Autodesk Inventor part; units mm, degrees
ref_plane "Work Plane2" through (0, 0, 16.5) normal (0, 0, 1) x (1, 0, 0)
ref_plane "YZ Plane" through (0, 0, 0) normal (1, 0, 0) x (0, 1, 0)
ref_plane "XZ Plane" through (0, 0, 0) normal (0, 1, 0) x (-1, 0, 0)
sketch "Sketch1" plane through (0, 0, 0) normal (0, 1, 0) x (-1, 0, 0)
  circle A0 centre (0, 0) radius 25
  dimension "d12" = 50
extrude "Extrusion1" add sketch "Sketch1" along normal blind 2
mirror "Mirror1" about plane through (0, 0, 0) normal (0, 0, 1)
ref_plane "Work Plane2" through (0, 0, 16.5) normal (0, 0, 1) x (1, 0, 0)
sketch "Sketch9" plane through (0, 0, 16.5) normal (0, 0, 1) x (1, 0, 0)
  line L0 (-5.099, 2) -> (5, 2)
  line L1 (5, 2) -> (5, 21)
  line L2 (-5.099, 20) -> (-5.099, 2)
  line L3 (0, -1.6) -> (0, 30.6) construction
  arc A0 (5, 21) -> (-5.099, 20) centre (0, 20) ccw
  circle A1 centre (0, 20) radius 1.9
  line L4 (25, 2) -> (-25, 2)
  dimension "d19" = 5
  dimension "d20" = 3.8
  dimension "d65" = 0
  dimension "d66" = 18
extrude "Extrusion3" add sketch "Sketch9" against normal blind 3
sketch "Sketch20" plane through (0, 0, 16.5) normal (0, 0, 1) x (1, 0, 0)
  circle A0 centre (0, 20) radius 1.9
  line L0 (-1.9, 20) -> (1.9, 20)
  line L1 (1.9, 20) -> (1.9, 25.4725)
  line L2 (1.9, 25.4725) -> (-1.9, 25.4725)
  line L3 (-1.9, 25.4725) -> (-1.9, 20)
  point P0 (0, 0)
extrude "Extrusion14" cut sketch "Sketch20" against normal blind 3 contours A0 L3 L2 L1
mirror "Mirror5" about plane through (0, 0, 0) normal (0, 0, 1) of "Extrusion3", "Extrusion14"
sketch "Sketch21" plane through (0, 0, 0) normal (0, -1, 0) x (1, 0, 0)
  circle A0 centre (0, 0) radius 16.95
  dimension "d62" = 33.9
extrude "Extrusion15" add sketch "Sketch21" along normal blind 30
ref_plane "Work Plane1" through (0, 0, 0) normal (0, 0, 1) x (1, 0, 0)
properties part number "BaseComple"
CAD build for the part. Positions are in the model's coordinates, mm. A direction names the side the tool comes from. Give positions to 0.01 mm unless a question says otherwise; leave off trailing zeros. Loops run counter-clockwise (first coordinate to the right, second up) from the corner with the lowest first, then second, coordinate; pieces in that order, holes last. Notation, with made-up numbers: (-32.75, 78) -> (-6.75, 78) arc R27 cw to (-6.75, 96) -> close; hole circle Ø11 at (40.5, 59). An arc over 180 degrees is marked (long way). Use a Markdown table: item, result.
1. Slice it at D-D (y = -22.5). List the corners of the cut face in (x, z).
Check result:
| item | result |
|---|---|
| outline | circle Ø33.9 at (0, 0) |
2. Flat gauge pins, fed straight in: pin 1 (2.5 mm diameter, centred on y = 8.5, z = 14.5, fed in from +X); pin 2 (0.9 mm diameter, centred on y = 22.5, z = 15.5, fed in from +X); pin 3 (10 mm diameter, centred on x = 12.5, z = -5, fed in from +Y). Where does each tip first touch, or does it go through?
Check result:
| item | result |
|---|---|
| pin 1 | stops at x = 5 |
| pin 2 | stops at x = 4.67 |
| pin 3 | stops at y = 2 |
3. Mould opens along Z. For faces 6 (the flat face through (-1.9, 22, 15)), 7 (the flat face through (0, 14, 16.5)), 8 (the flat face through (0, 14, 13.5)), 9 (the flat face through (0, 14, -16.5)) say: pulls with the +Z half, pulls with the -Z half, needs draft (parallel to the pull), parting line crosses it, or undercut.
Check result:
| item | result |
|---|---|
| face 6 | needs draft |
| face 7 | pulls with the +Z half |
| face 8 | undercut |
| face 9 | pulls with the -Z half |
4. Wall check: L1, parallel to Y at x = 19, z = -10.5; L2, parallel to Y at x = -8.5, z = -7; L3, parallel to X at y = 17, z = -14.5. Give the ranges that are in metal, low to high. Write a range as [from, to].
Check result:
| item | result |
|---|---|
| L1 | y = [0, 2] |
| L2 | y = [-30, 2] |
| L3 | x = [-5.1, 5] |
5. Slice it at C-C (x = -12.5). List the corners of the cut face in (y, z), plus the area to 3 significant figures.
Check result:
| item | result |
|---|---|
| outline | (-30, -11.45) -> (0, -11.45) -> (0, -21.65) -> (2, -21.65) -> (2, 21.65) -> (0, 21.65) -> (0, 11.45) -> (-30, 11.45) -> close |
| area | 773 mm^2 |
6. Which spindle directions (+Z, -Z, +X, -X, +Y, -Y) get a long thin tool onto all of the face, cutting with end or side? Do faces 1 (the cylindrical face through (-12.49, -14.79, -11.46)), 2 (the flat face through (5, 11, 15)), 3 (the flat face through (1.9, 22, -15)), 4 (the flat face through (-5.099, 11, -15)), 5 (the flat face through (0, -30, 0)). Say none if no direction does.
Check result:
| item | result |
|---|---|
| face 1 | -Y |
| face 2 | +Z, -Z, +X, +Y |
| face 3 | +Z, -Z, +Y |
| face 4 | +Z, -Z, -X, +Y |
| face 5 | +Z, -Z, +X, -X, -Y |
7. Slice it at B-B (x = 0). List the corners of the cut face in (y, z), plus the area to 3 significant figures.
Check result:
| item | result |
|---|---|
| outline | (-30, -16.95) -> (0, -16.95) -> (0, -25) -> (2, -25) -> (2, -16.5) -> (18.1, -16.5) -> (18.1, -13.5) -> (2, -13.5) -> (2, 13.5) -> (18.1, 13.5) -> (18.1, 16.5) -> (2, 16.5) -> (2, 25) -> (0, 25) -> (0, 16.95) -> (-30, 16.95) -> close |
| area | 1,210 mm^2 |
8. Slice it at A-A (y = 12.5). List the corners of the cut face in (x, z), plus the area to 3 significant figures.
Check result:
| item | result |
|---|---|
| outline | (-5.1, -16.5) -> (5, -16.5) -> (5, -13.5) -> (-5.1, -13.5) -> close; (-5.1, 13.5) -> (5, 13.5) -> (5, 16.5) -> (-5.1, 16.5) -> close |
| area | 60.6 mm^2 |
